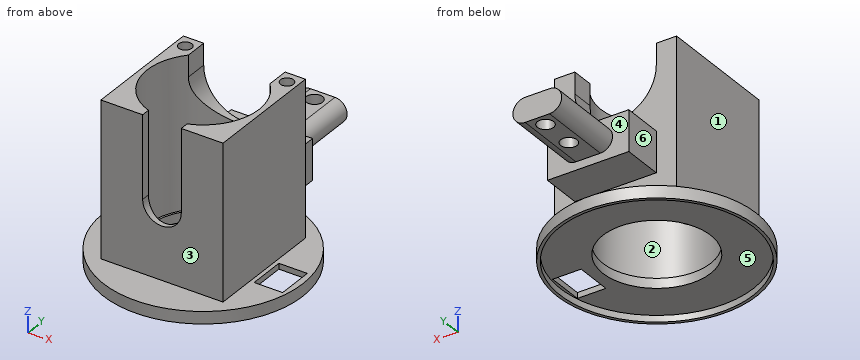
from build123d import *

# Parameters (mm, degrees)
SKETCH1_W                = 30
SKETCH1_H                = 30
BOSS_EXTRUDE1_DEPTH      = 38
CUT_EXTRUDE3_REACH       = 45.52
SKETCH2_R                = 13.25
SKETCH4_R                = 13.75
CUT_EXTRUDE4_DEPTH       = 37
SKETCH5_R                = 24.5
BOSS_EXTRUDE4_DEPTH      = 3
SKETCH8_R                = 23.75
CUT_EXTRUDE8_DEPTH       = 1.6
SKETCH9_R                = 13.25
CUT_EXTRUDE9_DEPTH       = 1.6
CUT_EXTRUDE10_REACH      = 53.425
SKETCH10_W               = 7
SKETCH10_H               = 9
CUT_EXTRUDE11_REACH      = 62.037
CUT_EXTRUDE11_END_RADIUS = 13.75
CUT_EXTRUDE12_REACH      = 62.037
CUT_EXTRUDE12_END_RADIUS = 13.75
SKETCH14_W               = 20
SKETCH14_H               = 10
BOSS_EXTRUDE5_DEPTH      = 10
BOSS_EXTRUDE6_DEPTH      = 18.5
CUT_EXTRUDE13_REACH      = 59.736
SKETCH16_R               = 2
SKETCH17_R               = 1.6
CUT_EXTRUDE14_DEPTH      = 10


with BuildPart() as part:
    # Sketch1 → Boss-Extrude1 (new body)
    with BuildSketch(Plane.XY):
        Rectangle(SKETCH1_W, SKETCH1_H)
    extrude(amount=BOSS_EXTRUDE1_DEPTH)

    # Sketch2 → Cut-Extrude3 (cut, up to next)
    with BuildSketch(Plane.XY.offset(38), mode=Mode.PRIVATE) as cut_extrude3_sk1:
        Circle(SKETCH2_R)
    cut_extrude3_tool1 = extrude(cut_extrude3_sk1.sketch, amount=-CUT_EXTRUDE3_REACH, mode=Mode.PRIVATE) & part.part
    add(cut_extrude3_tool1.solids().sort_by_distance((0, 0, 38))[0], mode=Mode.SUBTRACT)

    # Sketch4 → Cut-Extrude4 (cut)
    with BuildSketch(Plane.XY.offset(38)):
        Circle(SKETCH4_R)
    extrude(amount=-CUT_EXTRUDE4_DEPTH, mode=Mode.SUBTRACT)

    # Sketch5 → Boss-Extrude4 (add)
    with BuildSketch(Plane(origin=(0, 0, 0), x_dir=(-1, 0, 0), z_dir=(0, 0, -1))):
        Circle(SKETCH5_R)
    extrude(amount=BOSS_EXTRUDE4_DEPTH)

    # Sketch8 → Cut-Extrude8 (cut)
    with BuildSketch(Plane(origin=(0, 0, -3), x_dir=(-1, 0, 0), z_dir=(0, 0, -1))):
        Circle(SKETCH8_R)
    extrude(amount=-CUT_EXTRUDE8_DEPTH, mode=Mode.SUBTRACT)

    # Sketch9 → Cut-Extrude9 (cut)
    with BuildSketch(Plane.XY):
        Circle(SKETCH9_R)
    extrude(amount=-CUT_EXTRUDE9_DEPTH, mode=Mode.SUBTRACT)

    # Sketch10 → Cut-Extrude10 (cut, up to next)
    with BuildSketch(Plane.XY, mode=Mode.PRIVATE) as cut_extrude10_sk1:
        with Locations((19.5, -0.647719384)):
            Rectangle(SKETCH10_W, SKETCH10_H)
    cut_extrude10_tool1 = extrude(cut_extrude10_sk1.sketch, amount=-CUT_EXTRUDE10_REACH, mode=Mode.PRIVATE) & part.part
    add(cut_extrude10_tool1.solids().sort_by_distance((19.5, -0.647719, 0))[0], mode=Mode.SUBTRACT)

    # Cut-Extrude11: up to this cylinder (the profile starts outside it)
    cut_extrude11_end = Plane(origin=(0, 0, 27.875), z_dir=(0, 0, 1)) * Cylinder(CUT_EXTRUDE11_END_RADIUS, 152.574, mode=Mode.PRIVATE)
    # Sketch12 → Cut-Extrude11 (cut, up to the surface)
    with BuildSketch(Plane(origin=(0, -15, 0), x_dir=(-1, 0, 0), z_dir=(0, -1, 0)), mode=Mode.PRIVATE) as cut_extrude11_sk1:
        with BuildLine():
            Line((-4.75, -38), (-4.75, -17.75))
            ThreePointArc((-4.75, -17.75), (0, -13), (4.75, -17.75))
            Line((4.75, -17.75), (4.75, -38))
            ThreePointArc((4.75, -38), (0, -42.75), (-4.75, -38))
        make_face()
    cut_extrude11_tool1 = extrude(cut_extrude11_sk1.sketch, amount=-CUT_EXTRUDE11_REACH, mode=Mode.PRIVATE) - cut_extrude11_end
    add(cut_extrude11_tool1.solids().sort_by_distance((0, -15, 27.875))[0], mode=Mode.SUBTRACT)

    # Cut-Extrude12: up to this cylinder (the profile starts outside it)
    cut_extrude12_end = Plane(origin=(0, 0, 35.375), z_dir=(0, 0, 1)) * Cylinder(CUT_EXTRUDE12_END_RADIUS, 152.574, mode=Mode.PRIVATE)
    # Sketch13 → Cut-Extrude12 (cut, up to the surface)
    with BuildSketch(Plane(origin=(0, 15, 0), x_dir=(1, 0, 0), z_dir=(0, 1, 0)), mode=Mode.PRIVATE) as cut_extrude12_sk1:
        with BuildLine():
            Line((-10, -38), (-10, -32.75))
            ThreePointArc((-10, -32.75), (0, -22.75), (10, -32.75))
            Line((10, -32.75), (10, -38))
            ThreePointArc((10, -38), (0, -48), (-10, -38))
        make_face()
    cut_extrude12_tool1 = extrude(cut_extrude12_sk1.sketch, amount=-CUT_EXTRUDE12_REACH, mode=Mode.PRIVATE) - cut_extrude12_end
    add(cut_extrude12_tool1.solids().sort_by_distance((0, 15, 35.375))[0], mode=Mode.SUBTRACT)

    # Sketch14 → Boss-Extrude5 (add)
    with BuildSketch(Plane(origin=(0, 15, 0), x_dir=(1, 0, 0), z_dir=(0, 1, 0))):
        with Locations((0, -12)):
            Rectangle(SKETCH14_W, SKETCH14_H)
    extrude(amount=BOSS_EXTRUDE5_DEPTH)

    # Sketch15 → Boss-Extrude6 (add)
    with BuildSketch(Plane(origin=(0, 25, 0), x_dir=(1, 0, 0), z_dir=(0, 1, 0))):
        with BuildLine():
            Line((-3, -9), (3, -9))
            ThreePointArc((3, -9), (6, -12), (3, -15))
            Line((3, -15), (-3, -15))
            ThreePointArc((-3, -15), (-6, -12), (-3, -9))
        make_face()
    extrude(amount=BOSS_EXTRUDE6_DEPTH)

    # Sketch16 → Cut-Extrude13 (cut, up to next)
    with BuildSketch(Plane(origin=(0, 0, 9), x_dir=(-1, 0, 0), z_dir=(0, 0, -1)), mode=Mode.PRIVATE) as cut_extrude13_sk1:
        with Locations((0, 40.5)):
            Circle(SKETCH16_R)
    cut_extrude13_tool1 = extrude(cut_extrude13_sk1.sketch, amount=-CUT_EXTRUDE13_REACH, mode=Mode.PRIVATE) & part.part
    # Sketch16 → Cut-Extrude13 (cut, up to next)
    with BuildSketch(Plane(origin=(0, 0, 9), x_dir=(-1, 0, 0), z_dir=(0, 0, -1)), mode=Mode.PRIVATE) as cut_extrude13_sk2:
        with Locations((0, 32)):
            Circle(SKETCH16_R)
    cut_extrude13_tool2 = extrude(cut_extrude13_sk2.sketch, amount=-CUT_EXTRUDE13_REACH, mode=Mode.PRIVATE) & part.part
    add(cut_extrude13_tool1.solids().sort_by_distance((0, 40.5, 9))[0], mode=Mode.SUBTRACT)
    add(cut_extrude13_tool2.solids().sort_by_distance((0, 32, 9))[0], mode=Mode.SUBTRACT)

    # Sketch17 → Cut-Extrude14 (cut)
    with BuildSketch(Plane.XY.offset(38)):
        with Locations((12.5, 12)):
            Circle(SKETCH17_R)
        with Locations((-12.5, 12)):
            Circle(SKETCH17_R)
    extrude(amount=-CUT_EXTRUDE14_DEPTH, mode=Mode.SUBTRACT)


solid = part.part
Here's how the part is built. I have some questions about the finished solid (model axes, mm). Face numbers are marked on the shaded views. A direction names the side the tool comes from. Coordinates: 2 decimals unless noted, no trailing zeros. Order: outer loops, then holes, each group sorted by start corner. A loop starts at its lowest first (then second) coordinate and runs counter-clockwise, first axis right, second up.
Item 1: For the marked faces 1, 2 and 3, which set-ups out of +Z, -Z, +X, -X, +Y, -Y let a thin tool reach every point of the face, with its end or its side?
Result sheet:
face 1: +Z, -X, +Y, -Y
face 2: +Z
face 3: +Z, +X, -X, -Y
Item 2: If we section it at D-D on z = 2.5: List the corners of the cut face in (x, y) for me.
Result sheet:
outline: (-15, -15) - (15, -15) - (15, 15) - (-15, 15) - close; hole circle Ø27.5 at (0, 0)
Item 3: For P1, Ø5, axis at x = -1, y = 33, coming from the -Z side; P2, Ø1.8, axis at x = 1.5, y = 37.5, coming from the +Z side; P3, Ø0.7, axis at y = -1.5, z = -1, coming from the -X side, each with a flat end and sliding along its axis, tell me the tip position at first contact or that it passes through.
Result sheet:
P1: stops at z = 9
P2: stops at z = 15
P3: stops at x = -24.47
Item 4: If we section it at A-A on y = 32: List the corners of the cut face in (x, z) for me, plus the area to 3 significant figures.
Result sheet:
outline: (-3, 9) - (-2, 9) - (-2, 15) - (-3, 15) arc R3 ccw to start; (2, 9) - (3, 9) arc R3 ccw to (3, 15) - (2, 15) - close
area: 40.3 mm2
Item 5: If we section it at C-C on x = 8: List the corners of the cut face in (y, z) for me, plus the area to 3 significant figures.
Result sheet:
outline: (-23.16, -3) - (-22.36, -3) - (-22.36, -1.4) - (-10.56, -1.4) - (-10.56, 1) - (-11.18, 1) - (-11.18, 38) - (-15, 38) - (-15, 0) - (-23.16, 0) - close; (10.56, -1.4) - (22.36, -1.4) - (22.36, -3) - (23.16, -3) - (23.16, 0) - (15, 0) - (15, 7) - (25, 7) - (25, 17) - (15, 17) - (15, 26.75) - (11.18, 26.75) - (11.18, 1) - (10.56, 1) - close
area: 386 mm2
Item 6: If we mould it in two halves opening along Y, with no side actions, what happens to the marked faces 4, 5 and 6? For each: +Y half, -Y half, draft (parallel to the pull), parting line (faces both ways), or undercut.
Result sheet:
face 4: +Y half
face 5: undercut
face 6: draft
Item 7: If we section it at B-B on z = 12: List the corners of the cut face in (x, y) for me, plus the area to 3 significant figures.
Result sheet:
outline: (-15, -15) - (15, -15) - (15, 15) - (10, 15) - (10, 25) - (6, 25) - (6, 43.5) - (-6, 43.5) - (-6, 25) - (-10, 25) - (-10, 15) - (-15, 15) - close; hole circle Ø27.5 at (0, 0); hole circle Ø4 at (0, 32); hole circle Ø4 at (0, 40.5)
area: 703 mm2
Item 8: I need wall thicknesses on line 1 (X direction, y = 10, z = 36.5); line 2 (Y direction, x = 0, z = -2); line 3 (Y direction, x = 0, z = 12.6). Which ranges of each line are inside material? Lowest first, please.
Result sheet:
line 1: x = -15 to -10, 10 to 15
line 2: y = -24.5 to -23.75, 23.75 to 24.5
line 3: y = -15 to -13.75, 13.75 to 30, 34 to 38.5, 42.5 to 43.5
